```python
from build123d import *

# Parameters (mm, degrees)
SKETCH_W    = 60
SKETCH_H    = 48
SKETCH_R    = 2.5
SKETCH_R_2  = 6.5
PAD_DEPTH   = 10
FILLET_R    = 10
FILLET001_R = 1


with BuildPart() as part:
    # Sketch → Pad (new body)
    with BuildSketch(Plane.XY):
        with Locations((5, -91)):
            Rectangle(SKETCH_W, SKETCH_H)
        with Locations((25, -80)):
            Circle(SKETCH_R, mode=Mode.SUBTRACT)
        with Locations((-18, -80)):
            Circle(SKETCH_R, mode=Mode.SUBTRACT)
        with Locations((0, -85)):
            Circle(SKETCH_R_2, mode=Mode.SUBTRACT)
    extrude(amount=PAD_DEPTH)

    # Fillet
    fillet_edges = [part.edges().sort_by_distance(p)[0] for p in [
        (-25, -115, 5),
        (35, -115, 5),
    ]]
    fillet(fillet_edges, radius=FILLET_R)

    # Fillet001
    fillet001_edges = [part.edges().sort_by_distance(p)[0] for p in [
        (35, -67, 5),
        (-25, -67, 5),
    ]]
    fillet(fillet001_edges, radius=FILLET001_R)


solid = part.part
```
Can you work these out from the model? Positions are in its coordinate system, mm. Round coordinates to 2 decimals unless told otherwise and drop trailing zeros. Loops run counter-clockwise (first coordinate to the right, second up) from the corner with the lowest first, then second, coordinate; pieces in that order, holes last.
Item 1: If we mould it in two halves opening along X, with no side actions, what happens to faces 1 (the cylindrical face through (-20.5, -79.9, 4.9)), 2 (the flat face through (5, -91, 10)), 3 (the cylindrical face through (-22.15, -111.99, 5.07)), 4 (the cylindrical face through (-1.409, -91.345, 4.93))? For each: +X half, -X half, draft (parallel to the pull), parting line (faces both ways), or undercut.
Item 2: Please list where these lines run through material, in increasing order: L1, parallel to Y at x = 0, z = 7; L2, parallel to Y at x = -18, z = 4; L3, parallel to X at y = -89.5, z = 6.5.
Item 3: Suppose I cut it at D-D, the plane y = -80. Write out the boundary of the cut face in (x, z), then the cut area to 3 significant figures.
Item 4: Suppose I cut it at B-B, the plane y = -85. Write out the boundary of the cut face in (x, z).
Item 5: Suppose I cut it at A-A, the plane x = 0. Write out the boundary of the cut face in (y, z), then the cut area to 3 significant figures.
Item 6: Suppose I cut it at C-C, the plane z = 1.25. Write out the boundary of the cut face in (x, y), then the cut area to 3 significant figures.
Reported:
1. face 1: undercut
1. face 2: draft
1. face 3: -X half
1. face 4: undercut
2. L1: y = -115 to -91.5, -78.5 to -67
2. L2: y = -114.54 to -82.5, -77.5 to -67
2. L3: x = -25 to -4.69, 4.69 to 35
3. outline: (-25, 0) - (-20.5, 0) - (-20.5, 10) - (-25, 10) - close; (-15.5, 0) - (-4.15, 0) - (-4.15, 10) - (-15.5, 10) - close; (4.15, 0) - (22.5, 0) - (22.5, 10) - (4.15, 10) - close; (27.5, 0) - (35, 0) - (35, 10) - (27.5, 10) - close
3. area: 417 mm2
4. outline: (-25, 0) - (-6.5, 0) - (-6.5, 10) - (-25, 10) - close; (6.5, 0) - (35, 0) - (35, 10) - (6.5, 10) - close
5. outline: (-115, 0) - (-91.5, 0) - (-91.5, 10) - (-115, 10) - close; (-78.5, 0) - (-67, 0) - (-67, 10) - (-78.5, 10) - close
5. area: 350 mm2
6. outline: (-25, -105) arc R10 ccw to (-15, -115) - (25, -115) arc R10 ccw to (35, -105) - (35, -68) arc R1 ccw to (34, -67) - (-24, -67) arc R1 ccw to (-25, -68) - close; hole circle Ø5 at (-18, -80); hole circle Ø13 at (0, -85); hole circle Ø5 at (25, -80)
6. area: 2,660 mm2
